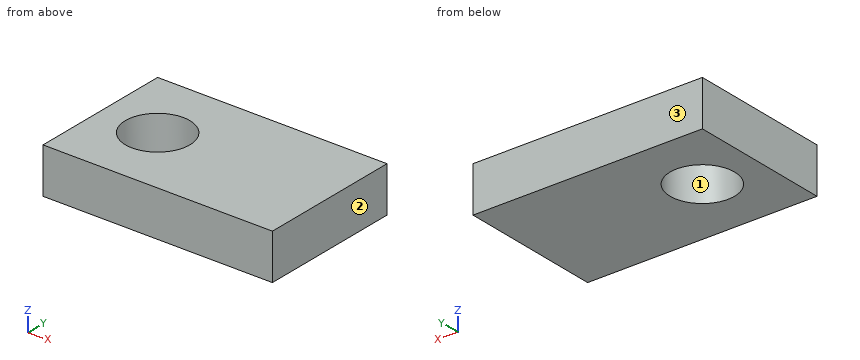
```python
from build123d import *

# Parameters (mm, degrees)
SKETCH1_W            = 16
SKETCH1_H            = 10
BOSS_EXTRUDE1_DEPTH  = 1.5875
M4_CLEARANCE_HOLE1_D = 4.5


with BuildPart() as part:
    # Sketch1 → Boss-Extrude1 (new body, symmetric)
    with BuildSketch(Plane.XY):
        Rectangle(SKETCH1_W, SKETCH1_H)
    extrude(amount=BOSS_EXTRUDE1_DEPTH, both=True)

    # M4 Clearance Hole1 (through all)
    with Locations(Plane.XY.offset(1.5875)):
        with Locations((-4, 0)):
            Hole(M4_CLEARANCE_HOLE1_D / 2)


solid = part.part
```
The model under review builds one solid part; all positions refer to its coordinate system, in mm. Face numbers are marked on the shaded views. Round coordinates to 2 decimals unless told otherwise and drop trailing zeros. Loops run counter-clockwise (first coordinate to the right, second up) from the corner with the lowest first, then second, coordinate; pieces in that order, holes last. Notation, with made-up numbers: (-34, -26.75) - (-5, -26.75) arc R21 cw to (-5, 7.25) - close; hole circle Ø10 at (71, 54.5). An arc over 180 degrees is marked (long way). Use a Markdown table: item, result. Add a question column.
Q1. Add section B-B (y = 0). State the section outline as (x, z) points.
Q2. Add section A-A (x = -4). State the section outline as (y, z) points.
Q3. The part is to be moulded in two halves that separate along X. For the marked faces 1, 2 and 3, say which applies: pulls with the +X half, pulls with the -X half, needs draft (parallel to the pull), parting line crosses it, or undercut.
Q4. Insertion check: pin 1 Ø6 at (x, y) = (-4, 0) entering from -Z. The pin has a flat end and moves straight along its axis. Give the tip position at first contact, or say it passes through.
Q5. For probe 1 along Y at (x, z) = (-4, 0.45); probe 2 along X at (y, z) = (-0.25, -1); probe 3 along X at (y, z) = (-1.25, 0.6), list the stretches that pass through material, from the lowest coordinate up.
Q6. Add section C-C (z = 0.55). State the section outline as (x, y) points.
Worked answers:
| question | item | result |
|---|---|---|
| 1 | outline | (-8, -1.59) - (-6.25, -1.59) - (-6.25, 1.59) - (-8, 1.59) - close; (-1.75, -1.59) - (8, -1.59) - (8, 1.59) - (-1.75, 1.59) - close |
| 2 | outline | (-5, -1.59) - (-2.25, -1.59) - (-2.25, 1.59) - (-5, 1.59) - close; (2.25, -1.59) - (5, -1.59) - (5, 1.59) - (2.25, 1.59) - close |
| 3 | face 1 | undercut |
| 3 | face 2 | pulls with the +X half |
| 3 | face 3 | needs draft |
| 4 | pin 1 | z = -1.59 |
| 5 | probe 1 | -5 to -2.25, 2.25 to 5 |
| 5 | probe 2 | -8 to -6.24, -1.76 to 8 |
| 5 | probe 3 | -8 to -5.87, -2.13 to 8 |
| 6 | outline | (-8, -5) - (8, -5) - (8, 5) - (-8, 5) - close; hole circle Ø4.5 at (-4, 0) |
